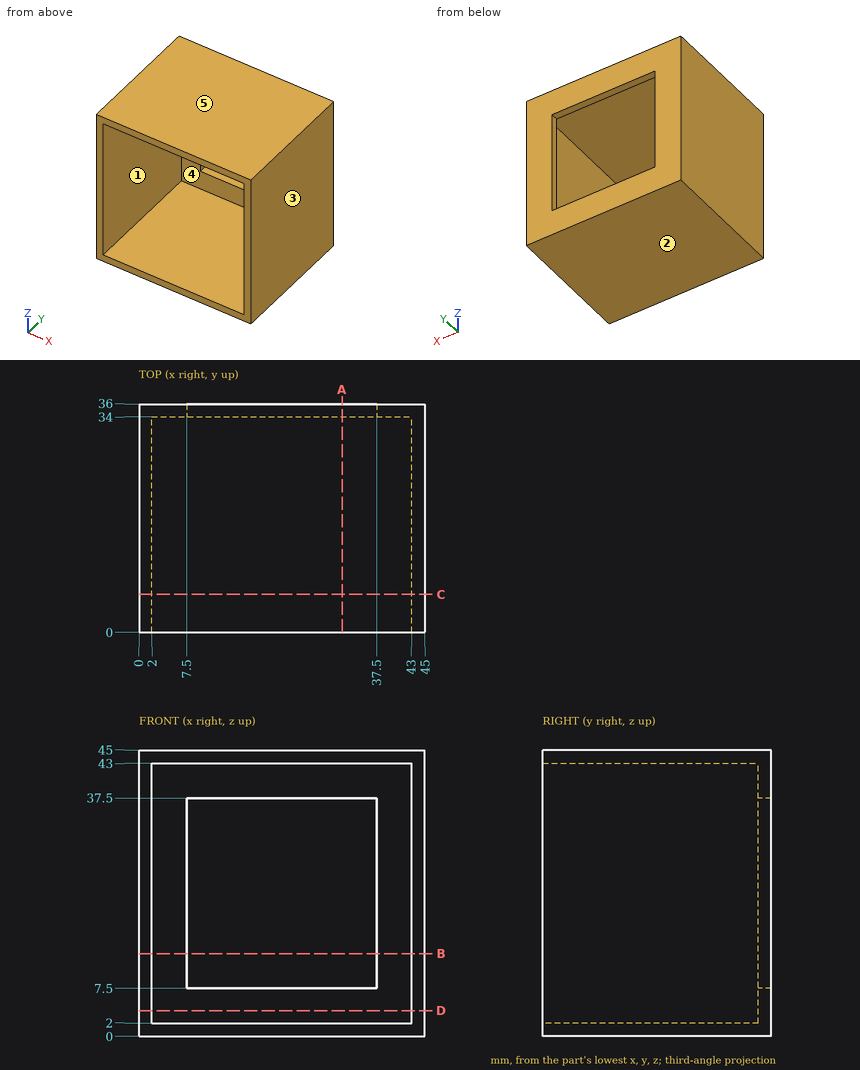
Print and shaded views of the part. All mm, measured from the part's lowest x, y and z. A direction names the side the tool comes from. Coordinates: 2 decimals unless noted, no trailing zeros. Loops run counter-clockwise (first coordinate to the right, second up) from the corner with the lowest first, then second, coordinate; pieces in that order, holes last. Notation, with made-up numbers: (-38, 61.25) - (6, 61.25) arc R21 cw to (6, 75.25) - close; hole circle Ø10 at (89, -28.5). An arc over 180 degrees is marked (long way). Write item = value, one per line. Start each with the question number.
Item 1: Saw through at D-D, the plane z = 4. List the corners of the cut face in (x, y), then the cut area to 3 significant figures.
Item 2: Wall check: probe 1 along X at (y, z) = (3, 35); probe 2 along Y at (x, z) = (19, 42.5). Give the ranges that are in metal, low to high. Write a range as [from, to].
Item 3: Saw through at C-C, the plane y = 6. List the corners of the cut face in (x, z).
Item 4: Saw through at B-B, the plane z = 13. List the corners of the cut face in (x, y).
Item 5: Pull direction X, two halves, no side cores. Call the marked faces 1, 2 and 3: +X half, -X half, draft (parallel to the pull), parting line (faces both ways), or undercut.
Item 6: 3-axis set-ups, long thin cutter, end or side, ignore diameter. For the marked faces 4 and 5: which of +Z, -Z, +X, -X, +Y, -Y reach the whole face in a straight line?
Item 7: Saw through at A-A, the plane x = 32. List the corners of the cut face in (y, z).
Answers:
q1.outline = (0, 0) - (2, 0) - (2, 34) - (43, 34) - (43, 0) - (45, 0) - (45, 36) - (0, 36) - close
q1.area = 226 mm2
q2.probe_1 = [0, 2], [43, 45]
q2.probe_2 = [34, 36]
q3.outline = (0, 0) - (45, 0) - (45, 45) - (0, 45) - close; hole (2, 2) - (43, 2) - (43, 43) - (2, 43) - close
q4.outline = (0, 0) - (2, 0) - (2, 34) - (7.5, 34) - (7.5, 36) - (0, 36) - close; (37.5, 34) - (43, 34) - (43, 0) - (45, 0) - (45, 36) - (37.5, 36) - close
q5.face_1 = undercut
q5.face_2 = draft
q5.face_3 = +X half
q6.face_4 = -Y
q6.face_5 = +Z, +X, -X, +Y, -Y
q7.outline = (0, 0) - (36, 0) - (36, 7.5) - (34, 7.5) - (34, 2) - (0, 2) - close; (0, 43) - (34, 43) - (34, 37.5) - (36, 37.5) - (36, 45) - (0, 45) - close
